Could you check a few things on this model? Use its own coordinates, in mm. A direction names the side the tool comes from. Give positions to 0.01 mm unless a question says otherwise; leave off trailing zeros. Loops run counter-clockwise (first coordinate to the right, second up) from the corner with the lowest first, then second, coordinate; pieces in that order, holes last. Notation, with made-up numbers: (40.25, 0) -> (97.25, 0) arc R25 cw to (97.25, 39) -> close; hole circle Ø10 at (62, 61). An arc over 180 degrees is marked (long way). Write item = value, one per line. Start each with the question number.
1) I want a section at C-C (z = 33.5). List the corners of the cut face in (x, y) for me, and give its area (3 significant figures).
2) If we mould it in two halves opening along Y, with no side actions, what happens to faces 1 (the face through (-17.824, -4.524, 17.49)), 2 (the face through (-63.29, -13.09, 31.53)), 3 (the face through (-50.763, -13, 31))? For each: +Y half, -Y half, draft (parallel to the pull), parting line (faces both ways), or undercut.
3) I want a section at B-B (x = -52). List the corners of the cut face in (y, z) for me, and give its area (3 significant figures).
4) On a 3-axis mill with a long thin cutter (end or side, diameter ignored), from which of +Z, -Z, +X, -X, +Y, -Y can I reach the whole of each face in a straight line? I mean faces 4 (the face through (-63, -22, 49.151)), 5 (the face through (-31.4, -15.3, 23.751)), 6 (the face through (-63, -19.031, 44)). Say none if no direction works.
5) I want a section at D-D (x = -31). List the corners of the cut face in (y, z) for me, and give its area (3 significant figures).
6) I want a section at A-A (z = 14). List the corners of the cut face in (x, y) for me, and give its area (3 significant figures).
7) I'm going to push flat-ended pins straight in: pin 1 Ø10 at (y, z) = (-21.5, 31) entering from +X; pin 2 Ø5.5 at (x, z) = (-66, 43) entering from +Y; pin 3 Ø12.5 at (x, y) = (-40, -15) entering from +Z; pin 4 Ø2 at (x, y) = (-68.5, -17) entering from +Z. Where does each tip first touch, or does it pass through?
8) I need wall thicknesses on probe 1 along Y at (x, z) = (-65, 37.5); probe 2 along Y at (x, z) = (-59.5, 45.5); probe 3 along X at (y, z) = (-18.5, 19). Which ranges of each line are inside material? Lowest first, please. Write a range as from..to.
from build123d import *

# Parameters (mm, degrees)
F1_DEPTH = 25.4
F3_DEPTH = 25.4
F4_R     = 6.35
F5_DEPTH = 25.4
F6_R     = 6.35
F7_DEPTH = 25.401
F9_DEPTH = 25.4


# Not quite as in the source:
# - ends of sketch curves that miss each other by under 0.0002 mm in the source are joined


with BuildPart() as f1:
    # F0 (on Front) → F1 (new body)
    with BuildSketch(Plane.XZ):
        Polygon((-76.163366437, 49.151442945), (-76.163366437, 11.051442945), (-12.663366437, 11.051442945), (-12.663366437, 23.751442945), (-50.763366437, 23.751442945), (-50.763366437, 49.151442945), align=None)
    extrude(amount=F1_DEPTH)

    # F2 (on face) → F3 (cut)
    with BuildSketch(Plane.XY.offset(23.751442945)):
        with BuildLine():
            ThreePointArc((-26.0716341436, 0), (-17.7255959226, -4.6165280857), (-12.663366437, -12.7))
            Line((-12.663366437, -12.7), (-12.663366437, 0))
            Line((-12.663366437, 0), (-26.0716341436, 0))
        make_face()
        with BuildLine():
            Line((-12.663366437, -25.4), (-12.663366437, -12.7))
            ThreePointArc((-12.663366437, -12.7), (-17.065136592, -20.482800112), (-24.5329812169, -25.4))
            Line((-24.5329812169, -25.4), (-12.663366437, -25.4))
        make_face()
    extrude(amount=-F3_DEPTH, mode=Mode.SUBTRACT)

    # F4 (on face) → F5 (cut)
    with BuildSketch(Plane.XY.offset(23.751442945)):
        with BuildLine():
            ThreePointArc((-19.0133373642, -12.7271744008), (-25.3531445932, -6.3771825813), (-31.7133046421, -12.7067888852))
            ThreePointArc((-31.7133046421, -12.7067888852), (-25.3735301351, -19.0771662202), (-19.0133373642, -12.7271744008))
        make_face()
        with Locations((-38.0633682514, -12.706788681)):
            Circle(F4_R)
    extrude(amount=-F5_DEPTH, mode=Mode.SUBTRACT)

    # F6 (on face) → F7 (cut, through all)
    with BuildSketch(Plane.YZ.offset(-50.763366437)):
        with Locations((-12.7, 37.8679819405)):
            Circle(F6_R)
    extrude(amount=-F7_DEPTH, mode=Mode.SUBTRACT)

    # F8 (on face) → F9 (cut)
    with BuildSketch(Plane.YZ.offset(-50.763366437)):
        with BuildLine():
            Line((-19.0313366339, 49.151442945), (-19.0313366339, 38.3544759569))
            ThreePointArc((-19.0313366339, 38.3544759569), (-12.456574062, 44.2133143835), (-6.35, 37.8679819405))
            Line((-6.35, 37.8679819405), (-6.3313366339, 49.151442945))
            Line((-6.3313366339, 49.151442945), (-19.0313366339, 49.151442945))
        make_face()
    extrude(amount=-F9_DEPTH, mode=Mode.SUBTRACT)


solid = f1.part
Answer list:
q1.outline = (-76.16, -25.4) -> (-50.76, -25.4) -> (-50.76, -17.31) -> (-76.16, -17.31) -> close; (-76.16, -8.09) -> (-50.76, -8.09) -> (-50.76, 0) -> (-76.16, 0) -> close
q1.area = 411 mm^2
q2.face_1 = +Y half
q2.face_2 = undercut
q2.face_3 = draft
q3.outline = (-25.4, 11.05) -> (0, 11.05) -> (0, 49.15) -> (-6.33, 49.15) -> (-6.35, 37.87) arc R6.35 cw (long way) to (-19.03, 38.35) -> (-19.03, 49.15) -> (-25.4, 49.15) -> close
q3.area = 761 mm^2
q4.face_4 = +Z, +X, -X, +Y, -Y
q4.face_5 = +Z, +X, +Y, -Y
q4.face_6 = +Z, +X, -X
q5.outline = (-25.4, 11.05) -> (-15.65, 11.05) -> (-15.65, 23.75) -> (-25.4, 23.75) -> close; (-9.8, 11.05) -> (0, 11.05) -> (0, 23.75) -> (-9.8, 23.75) -> close
q5.area = 248 mm^2
q6.outline = (-76.16, -25.4) -> (-24.53, -25.4) arc R19.05 ccw to (-12.66, -12.7) arc R19.05 ccw to (-26.07, 0) -> (-76.16, 0) -> close; hole circle Ø12.7 at (-38.06, -12.71); hole circle Ø12.7 at (-25.36, -12.73)
q6.area = 1,250 mm^2
q7.pin_1 = -50.76
q7.pin_2 = 0
q7.pin_3 = 23.75
q7.pin_4 = 34.37
q8.probe_1 = -25.4..-19.04, -6.36..0
q8.probe_2 = -25.4..-19.03, -6.34..0
q8.probe_3 = -76.16..-40.66, -35.46..-28.01, -22.72..-15.45
